Could you check a few things on this model? Use its own coordinates, in mm. Face numbers are marked on the shaded views. A direction names the side the tool comes from. Give positions to 0.01 mm unless a question says otherwise; leave off trailing zeros. Order: outer loops, then holes, each group sorted by start corner. A loop starts at its lowest first (then second) coordinate and runs counter-clockwise, first axis right, second up. Notation, with made-up numbers: (70, -40) - (129, -40) arc R16 ccw to (129, -24) - close; hole circle Ø1 at (-7.75, 14). An arc over 180 degrees is marked (long way). Put each result on its own line as item: value.
from build123d import *

# Parameters (mm, degrees)
EXTRUDE_1_DEPTH          = 48
CUT_EXTRUDE_1_DEPTH      = 60.304300013
CUT_EXTRUDE_1_DEPTH_BACK = 60.304300013
SKETCH_3_R               = 4
CUT_EXTRUDE_2_DEPTH      = 60.304300013
CUT_EXTRUDE_2_DEPTH_BACK = 60.304300013
SKETCH_4_R               = 4
SKETCH_5_W               = 48
SKETCH_5_H               = 4
EXTRUDE_3_DEPTH          = 12
CUT_EXTRUDE_3_DEPTH      = 66.39217114
CUT_EXTRUDE_3_DEPTH_BACK = 25
CUT_EXTRUDE_3_START      = 15
SKETCH_7_R               = 1.45
CUT_EXTRUDE_4_DEPTH      = 66.39217114
CUT_EXTRUDE_4_DEPTH_BACK = 66.39217114
CUT_EXTRUDE_5_DEPTH      = 8
SKETCH_10_R              = 1.5
CUT_EXTRUDE_6_DEPTH      = 10
SKETCH_11_W              = 5.6
SKETCH_11_H              = 2.8
CUT_EXTRUDE_7_DEPTH      = 10
SKETCH_13_R              = 1.5
EXTRUDE_4_DEPTH          = 9.5
FILLET_2_R               = 15
FILLET_4_R               = 8
FILLET_5_R               = 2
EXTRUDE_5_DEPTH          = 6
FILLET_6_R               = 2
FILLET_7_R               = 1
EXTRUDE_START            = -9
SKETCH_15_W              = 3
SKETCH_15_H              = 14
EXTRUDE_6_DEPTH          = 6
FILLET_8_R               = 3
SKETCH_16_W              = 5.6
SKETCH_16_H              = 2.8
CUT_EXTRUDE_8_DEPTH      = 7
CUT_EXTRUDE_9_DEPTH      = 2.5
CUT_EXTRUDE_9_DRAFT      = -5


# Some blends are built 0.0001 mm under size
with BuildPart() as part:
    # Эскиз2 → Бобышка-Вытянуть1 (new body)
    with BuildSketch(Plane.XY):
        with BuildLine():
            Line((0.5, -7.483314774), (0.5, -10.988630488))
            ThreePointArc((0.5, -10.988630488), (7.95298686, -7.599342077), (11, 0))
            Line((11, 0), (11, 27))
            Line((11, 27), (-11, 27))
            Line((-11, 27), (-11, 0))
            ThreePointArc((-11, 0), (-7.95298686, -7.599342077), (-0.5, -10.988630488))
            Line((-0.5, -10.988630488), (-0.5, -7.483314774))
            ThreePointArc((-0.5, -7.483314774), (0, 7.5), (0.5, -7.483314774))
        make_face()
    extrude(amount=EXTRUDE_1_DEPTH)

    # Эскиз3 → Вырез-Вытянуть1 (cut, two sides: drawn at the far end of the back side and taken through both)
    with BuildSketch(Plane(origin=(11, 0, 0), x_dir=(0, 0, -1), z_dir=(1, 0, 0)).offset(-CUT_EXTRUDE_1_DEPTH_BACK)):
        with Locations((-40, 12)):
            Circle(SKETCH_3_R)
    extrude(amount=CUT_EXTRUDE_1_DEPTH + CUT_EXTRUDE_1_DEPTH_BACK, mode=Mode.SUBTRACT)

    # Эскиз4 → Вырез-Вытянуть2 (cut, two sides: drawn at the far end of the back side and taken through both)
    with BuildSketch(Plane(origin=(11, 0, 0), x_dir=(0, 0, -1), z_dir=(1, 0, 0)).offset(-CUT_EXTRUDE_2_DEPTH_BACK)):
        with Locations((-8, 12)):
            Circle(SKETCH_4_R)
    extrude(amount=CUT_EXTRUDE_2_DEPTH + CUT_EXTRUDE_2_DEPTH_BACK, mode=Mode.SUBTRACT)

    # Эскиз5 → Бобышка-Вытянуть3 (add)
    with BuildSketch(Plane(origin=(11, 0, 0), x_dir=(0, 0, -1), z_dir=(1, 0, 0))):
        with Locations((-24, 25)):
            Rectangle(SKETCH_5_W, SKETCH_5_H)
    extrude(amount=EXTRUDE_3_DEPTH)

    # Эскиз7 → Вырез-Вытянуть3 (cut, two sides: drawn at the far end of the back side and taken through both)
    with BuildSketch(Plane(origin=(0, 27, 0), x_dir=(1, 0, 0), z_dir=(0, 1, 0)).offset(CUT_EXTRUDE_3_START - CUT_EXTRUDE_3_DEPTH_BACK)):
        with Locations(Location((8, -35, 0), (0, 0, 270))):
            Circle(SKETCH_7_R)
        with Locations(Location((18.5, -13, 0), (0, 0, 270))):
            Circle(SKETCH_7_R)
    extrude(amount=CUT_EXTRUDE_3_DEPTH + CUT_EXTRUDE_3_DEPTH_BACK, mode=Mode.SUBTRACT)

    # Эскиз8 → Вырез-Вытянуть4 (cut, two sides: drawn at the far end of the back side and taken through both)
    with BuildSketch(Plane(origin=(0, 27, 0), x_dir=(1, 0, 0), z_dir=(0, 1, 0)).offset(-CUT_EXTRUDE_4_DEPTH_BACK)):
        with BuildLine():
            Line((23, -48), (20, -48))
            ThreePointArc((20, -48), (22.121320344, -47.121320344), (23, -45))
            Line((23, -45), (23, -48))
        make_face()
        with BuildLine():
            Line((23, 0), (23, -3))
            ThreePointArc((23, -3), (22.121320344, -0.878679656), (20, 0))
            Line((20, 0), (23, 0))
        make_face()
    extrude(amount=CUT_EXTRUDE_4_DEPTH + CUT_EXTRUDE_4_DEPTH_BACK, mode=Mode.SUBTRACT)

    # Эскиз9 → Вырез-Вытянуть5 (cut)
    with BuildSketch(Plane(origin=(0, 27, 0), x_dir=(1, 0, 0), z_dir=(0, 1, 0))):
        Polygon((-11, -48), (23, -48), (23, -40), (0, -40), (0, -8), (23, -8), (23, 0), (-11, 0), (-11, -8), (-11, -40), align=None)
    extrude(amount=-CUT_EXTRUDE_5_DEPTH, mode=Mode.SUBTRACT)

    # Эскиз10 → Вырез-Вытянуть6 (cut)
    with BuildSketch(Plane(origin=(0, 19, 0), x_dir=(1, 0, 0), z_dir=(0, 1, 0))):
        with Locations(Location((-5.5, -24, 0), (0, 0, 270))):
            Circle(SKETCH_10_R)
    extrude(amount=-CUT_EXTRUDE_6_DEPTH, mode=Mode.SUBTRACT)

    # Эскиз11 → Вырез-Вытянуть7 (cut)
    with BuildSketch(Plane.ZY.offset(11)):
        with Locations((24, 12.6)):
            Rectangle(SKETCH_11_W, SKETCH_11_H)
    extrude(amount=-CUT_EXTRUDE_7_DEPTH, mode=Mode.SUBTRACT)

    # Эскиз13 → Бобышка-Вытянуть4 (add)
    with BuildSketch(Plane(origin=(0, 27, 0), x_dir=(1, 0, 0), z_dir=(0, 1, 0))):
        with BuildLine():
            Line((21, -8), (13.5, -8))
            ThreePointArc((13.5, -8), (12.085786438, -8.585786438), (11.5, -10))
            Line((11.5, -10), (11.5, -22))
            ThreePointArc((11.5, -22), (12.085786438, -23.414213562), (13.5, -24))
            Line((13.5, -24), (21, -24))
            ThreePointArc((21, -24), (22.414213562, -23.414213562), (23, -22))
            Line((23, -22), (23, -10))
            Line((23, -10), (23, -8))
            Line((23, -8), (21, -8))
        make_face()
        with Locations(Location((18.5, -13, 0), (0, 0, 270))):
            Circle(SKETCH_13_R, mode=Mode.SUBTRACT)
    extrude(amount=EXTRUDE_4_DEPTH)

    # Скругление2
    # the kernel refuses this fillet: 15 mm, written as the material it takes off along each edge
    with BuildSketch(Plane(origin=(23, 64.5, 40), x_dir=(-1, 0, 0), z_dir=(0, -1, 0))) as fillet_2_piece_1_section:
        with BuildLine():
            CenterArc((FILLET_2_R, FILLET_2_R), FILLET_2_R, 180, 90)
            Line((0, FILLET_2_R), (0, 0))
            Line((0, 0), (FILLET_2_R, 0))
        make_face()
    fillet_2_piece_1 = extrude(amount=79, mode=Mode.PRIVATE)
    fillet_2_piece_1 = split(fillet_2_piece_1, bisect_by=Plane(origin=(10.251523637, 19, 39.909241185), z_dir=(0, 1, 0)), keep=Keep.TOP, mode=Mode.PRIVATE)
    add(fillet_2_piece_1, mode=Mode.SUBTRACT)

    # Скругление4
    fillet_4_edges = [part.edges().sort_by_distance(p)[0] for p in [
        (0, 19, 48),
        (0, 19, 0),
    ]]
    fillet(fillet_4_edges, radius=FILLET_4_R - 0.0001)  # a hair under: the kernel refuses the full size

    # Скругление5
    fillet_5_edges = [part.edges().sort_by_distance(p)[0] for p in [
        (23, 23, 16.5),
        (19.618950039, 23, 34.486832981),
    ]]
    fillet(fillet_5_edges, radius=FILLET_5_R)

    # Эскиз14 → Бобышка-Вытянуть5 (add)
    with BuildSketch(Plane(origin=(0, 0, 8), x_dir=(-1, 0, 0), z_dir=(0, 0, -1))):
        with BuildLine():
            Line((-23, 36.5), (-18.933112149, 36.5))
            Line((-18.933112149, 36.5), (-18.933112149, 23))
            Line((-18.933112149, 23), (-21, 23))
            ThreePointArc((-21, 23), (-22.414213562, 23.585786438), (-23, 25))
            Line((-23, 25), (-23, 36.5))
        make_face()
    extrude(amount=EXTRUDE_5_DEPTH)

    # Скругление6
    fillet_6_edges = [part.edges().sort_by_distance(p)[0] for p in [
        (18.933112149, 29.75, 8),
    ]]
    fillet(fillet_6_edges, radius=FILLET_6_R)

    # Скругление7
    fillet_7_edges = [part.edges().sort_by_distance(p)[0] for p in [
        (18.933112149, 29.75, 2),
    ]]
    fillet(fillet_7_edges, radius=FILLET_7_R)

    # Эскиз15 → Бобышка-Вытянуть6 (add)
    with BuildSketch(Plane(origin=(0, 0, 0), x_dir=(-1, 0, 0), z_dir=(0, 0, -1)).offset(EXTRUDE_START)):
        with Locations((2, -14.483314774)):
            Rectangle(SKETCH_15_W, SKETCH_15_H)
    extrude(amount=-EXTRUDE_6_DEPTH)

    # Скругление8
    fillet_8_edges = [part.edges().sort_by_distance(p)[0] for p in [
        (-2, -21.483314774, 15),
    ]]
    fillet(fillet_8_edges, radius=FILLET_8_R)

    # Эскиз16 → Вырез-Вытянуть8 (cut)
    with BuildSketch(Plane(origin=(11, 0, 0), x_dir=(0, 0, -1), z_dir=(1, 0, 0))):
        with Locations((-35, 18.4)):
            Rectangle(SKETCH_16_W, SKETCH_16_H)
    extrude(amount=-CUT_EXTRUDE_8_DEPTH, mode=Mode.SUBTRACT)


with BuildPart() as cut_extrude_9_tool:
    # Эскиз19 → Вырез-Вытянуть9 (with draft: the straight prism first)
    with BuildSketch(Plane.XZ.offset(-23)):
        Polygon((18.5, 16.175426481), (15.75, 14.58771324), (15.75, 11.41228676), (18.5, 9.824573519), (21.25, 11.41228676), (21.25, 14.58771324), align=None)
    extrude(amount=-CUT_EXTRUDE_9_DEPTH)
    # Вырез-Вытянуть9: the draft: its side faces are tilted about the plane it starts from
    cut_extrude_9_sides = [cut_extrude_9_tool.faces().sort_by_distance(p)[0] for p in [
        (17.125, 24.25, 15.38156986),
        (15.75, 24.25, 13),
        (17.125, 24.25, 10.61843014),
        (19.875, 24.25, 10.61843014),
        (21.25, 24.25, 13),
        (19.875, 24.25, 15.38156986),
    ]]
    draft(cut_extrude_9_sides, Plane.XZ.offset(-23), CUT_EXTRUDE_9_DRAFT)


with BuildPart() as part_1:
    add(part.part)

    # Вырез-Вытянуть9: cut by cut_extrude_9_tool
    add(cut_extrude_9_tool.part, mode=Mode.SUBTRACT)


solid = part_1.part
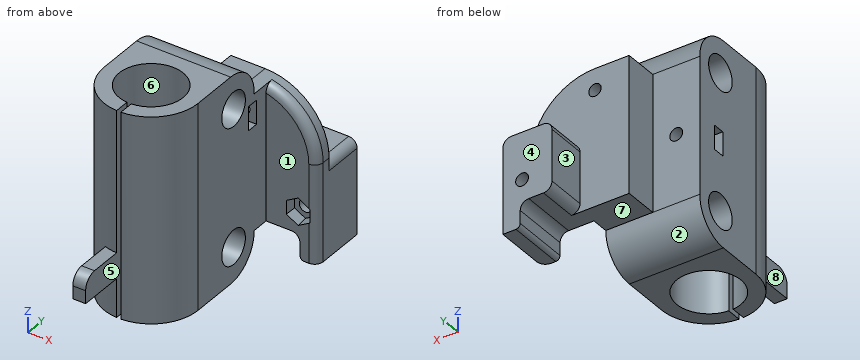
1) Which directions (+Z, -Z, +X, -X, +Y, -Y) give clear straight access to the entire face, cutting with the end or side of a thin tool? Please do the marked faces 1, 2, 3, 4 and 5.
Filled in:
face 1: +Z, -Z, +X, -Y
face 2: -Z, +X, -X, +Y
face 3: +Z, -Z, -X, +Y
face 4: +Z, -Z, +X, -X, +Y
face 5: +Z, -Z, -Y
2) Suppose I cut it at D-D, the plane y = 12. List the corners of the cut face in (x, z) for me.
Filled in:
outline: (-11, 0.06) - (11, 0.06) - (11, 4) - (-11, 4) - close; (-11, 12) - (11, 12) - (11, 36) - (-11, 36) - (-11, 26.8) - (-1, 26.8) - (-1, 21.2) - (-11, 21.2) - close; (-11, 44) - (11, 44) - (11, 47.94) - (-11, 47.94) - close
3) I'm going to push flat-ended pins straight in: pin 1 (3 mm diameter, centred on x = 6, z = 35, fed in from +Y); pin 2 (3 mm diameter, centred on x = 12, y = 25, fed in from -Z); pin 3 (9 mm diameter, centred on y = 12, z = 8, fed in from -X); pin 4 (6.5 mm diameter, centred on y = -16, z = 11.5, fed in from -X). Where does each tip first touch, or does it pass through?
Filled in:
pin 1: stops at y = 27
pin 2: stops at z = 8
pin 3: stops at x = -11
pin 4: stops at x = -3.5
4) Suppose I cut it at C-C, the plane y = 28.5. List the corners of the cut face in (x, z) for me, and give its area (3 significant figures).
Filled in:
outline: (11.5, 10) arc R2 ccw to (13.5, 8) - (16.93, 8) arc R2 cw to (18.93, 6) - (18.93, 3) arc R1 ccw to (19.93, 2) - (23, 2) - (23, 22) arc R2 ccw to (21, 24) - (13.5, 24) arc R2 ccw to (11.5, 22) - close; hole circle Ø3 at (18.5, 13)
area: 199 mm^2
5) Suppose I cut it at A-A, the plane y = 6. List the corners of the cut face in (x, z) for me, and give its area (3 significant figures).
Filled in:
outline: (-11, 0) - (-4.5, 0) - (-4.5, 48) - (-11, 48) - close; (4.5, 0) - (11, 0) - (11, 48) - (4.5, 48) - close
area: 624 mm^2
6) Suppose I cut it at B-B, the plane x = -5.5. List the corners of the cut face in (y, z) for me, and give its area (3 significant figures).
Filled in:
outline: (-9.53, 0) - (-5.1, 0) - (-5.1, 48) - (-9.53, 48) - close; (5.1, 0) - (11, 0) arc R8 ccw to (19, 8) - (19, 22.5) - (14, 22.5) - (14, 21.2) - (11.2, 21.2) - (11.2, 22.5) - (9, 22.5) - (9, 25.5) - (11.2, 25.5) - (11.2, 26.8) - (14, 26.8) - (14, 25.5) - (19, 25.5) - (19, 40) arc R8 ccw to (11, 48) - (5.1, 48) - close; hole circle Ø8 at (12, 8); hole circle Ø8 at (12, 40)
area: 714 mm^2
7) If I drill on line 1 (X direction, y = 0, z = 38); line 2 (Z direction, x = 6.5, y = 13); line 3 (X direction, y = 10.55, z = 24), over which ranges is the centre line in solid material (lowest first)? Write a range as [from, to].
Filled in:
line 1: x = [-11, -7.5], [7.5, 11]
line 2: z = [0.25, 4.13], [11.87, 36.13], [43.87, 47.75]
line 3: x = [-11, -7], [-4, 11]
8) We'd pull the mould along X, two halves only. Please class the marked faces 6, 7 and 8: pulls with the +X half, pulls with the -X half, needs draft (parallel to the pull), parting line crosses it, or undercut.
Filled in:
face 6: undercut
face 7: needs draft
face 8: pulls with the -X half
